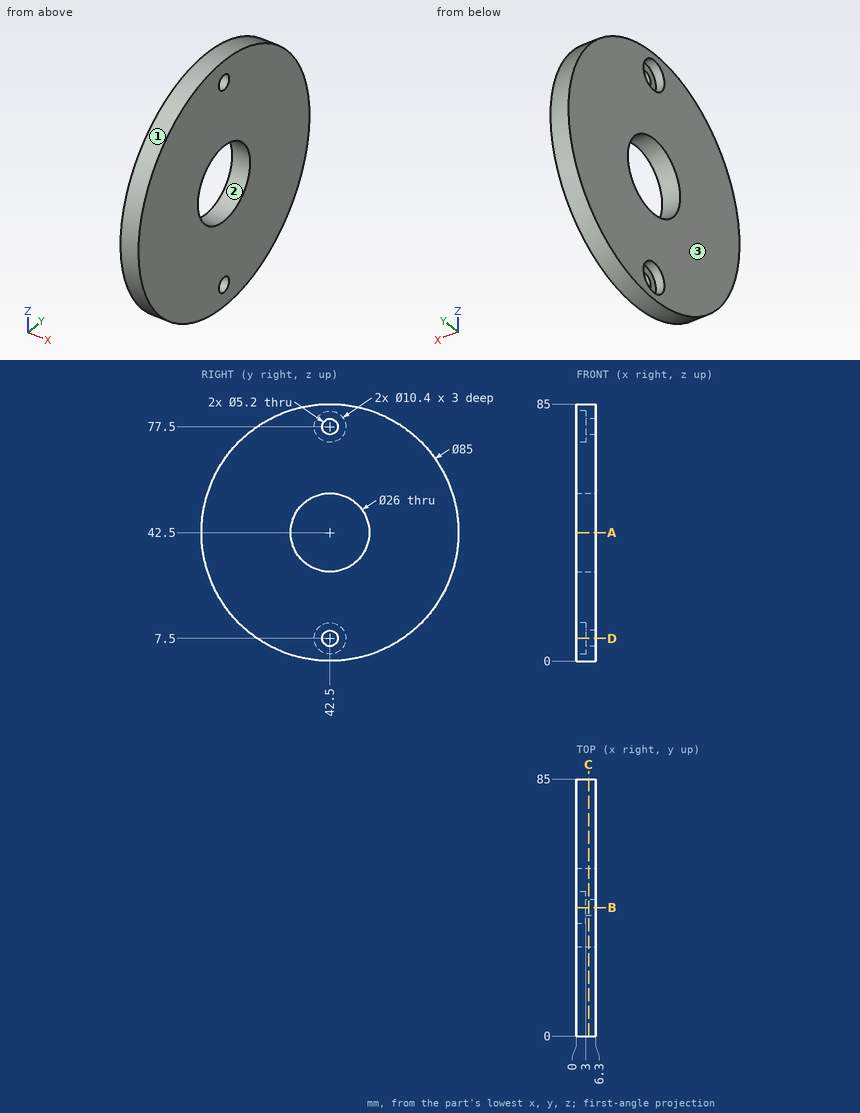
Geometry check sheet. Reference: drawing and pictorial views, mm from the part's lowest x, y, z. Round coordinates to 2 decimals unless told otherwise and drop trailing zeros. Write each loop counter-clockwise with the first axis right and the second up, starting at its lowest first coordinate (ties: lowest second). Pieces come first, ordered by that corner, then holes.
Item 1: Section check D-D (z = 7.5). Record the boundary of the cut face in (x, y).
Determined:
outline: (0, 18.39) - (6.3, 18.39) - (6.3, 39.9) - (3, 39.9) - (3, 37.3) - (0, 37.3) - close; (0, 47.7) - (3, 47.7) - (3, 45.1) - (6.3, 45.1) - (6.3, 66.61) - (0, 66.61) - close
Item 2: Section check B-B (y = 42.5). Record the boundary of the cut face in (x, z).
Determined:
outline: (0, 0) - (6.3, 0) - (6.3, 4.9) - (3, 4.9) - (3, 2.3) - (0, 2.3) - close; (0, 12.7) - (3, 12.7) - (3, 10.1) - (6.3, 10.1) - (6.3, 29.5) - (0, 29.5) - close; (0, 55.5) - (6.3, 55.5) - (6.3, 74.9) - (3, 74.9) - (3, 72.3) - (0, 72.3) - close; (0, 82.7) - (3, 82.7) - (3, 80.1) - (6.3, 80.1) - (6.3, 85) - (0, 85) - close
Item 3: Material ranges on line 1 along Z through (x, y) = (0.5, 32.5); line 2 along Y through (x, z) = (3.75, 70); line 3 along Y through (x, z) = (0.5, 36), recorded low to high.
Determined:
line 1: z = 1.19 to 34.19, 50.81 to 83.81
line 2: y = 10.1 to 74.9
line 3: y = 0.5 to 31.24, 53.76 to 84.5
Item 4: Go/stop test with flat-tipped pins: pin 1 Ø8.5 at (y, z) = (42.5, 7.5) entering from -X; pin 2 Ø2 at (x, z) = (4.5, 64.5) entering from -Y; pin 3 Ø3 at (x, y) = (2, 34.5) entering from -Z. Record where each tip stops, or that it passes through.
Determined:
pin 1: stops at x = 3
pin 2: stops at y = 5.55
pin 3: stops at z = 0.5
Item 5: Section check C-C (x = 4). Record the boundary of the cut face in (y, z), plus the area to 3 significant figures.
Determined:
outline: circle Ø85 at (42.5, 42.5); hole circle Ø26 at (42.5, 42.5); hole circle Ø5.2 at (42.5, 7.5); hole circle Ø5.2 at (42.5, 77.5)
area: 5,100 mm2
Item 6: Mould release check, pull along Z, two halves, no side actions. Record for the marked faces 1, 2 and 3: +Z half, -Z half, draft (parallel to the pull), parting line (faces both ways), or undercut.
Determined:
face 1: parting line
face 2: undercut
face 3: draft
Item 7: Section check A-A (z = 42.5). Record the boundary of the cut face in (x, y), plus the area to 3 significant figures.
Determined:
outline: (0, 0) - (6.3, 0) - (6.3, 29.5) - (0, 29.5) - close; (0, 55.5) - (6.3, 55.5) - (6.3, 85) - (0, 85) - close
area: 372 mm2
